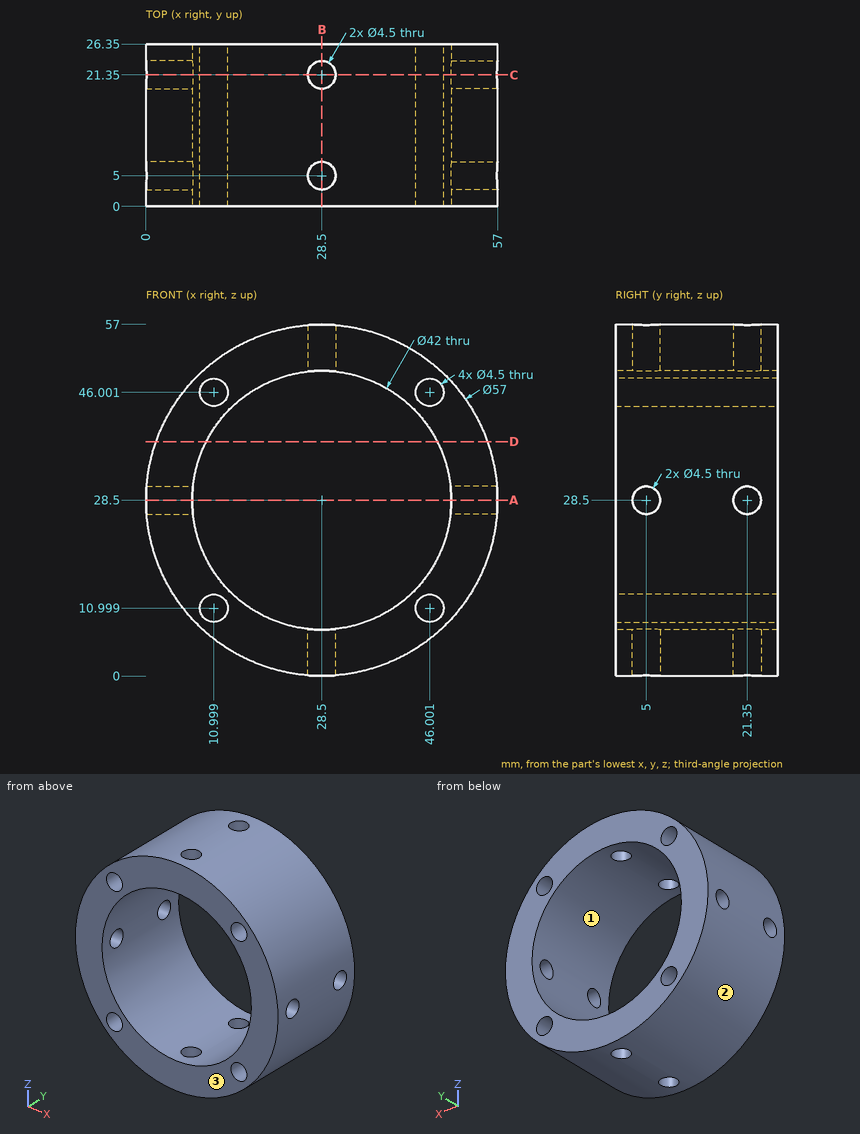
Here's the drawing with two shaded views (mm, measured from the low corner). I have some questions. Give positions to 0.01 mm unless a question says otherwise; leave off trailing zeros. Loops run counter-clockwise (first coordinate to the right, second up) from the corner with the lowest first, then second, coordinate; pieces in that order, holes last. Notation, with made-up numbers: M -17,35.25 L 6,35.25 A31 cw 6,70.25 Z; hole C -36.5,77.5 d1. An arc over 180 degrees is marked long. Use one line per item in the form item = value. Start each with the question number.
Q1. If we section it at B-B (x = 28.5): Write out the boundary of the cut face in (y, z).
Q2. If we section it at D-D (z = 38): Write out the boundary of the cut face in (x, y).
Q3. Will these pins go through, and if not, where does the flat tip stop? pin 1 Ø4 at (x, y) = (28.5, 5) entering from -Z; pin 2 Ø8 at (y, z) = (6, 8.5) entering from +X (3 decimals); pin 3 Ø1 at (x, y) = (37.5, 13) entering from +Z; pin 4 Ø1.5 at (x, y) = (47, 5) entering from -Z.
Q4. If we section it at C-C (y = 21.35): Write out the boundary of the cut face in (x, z).
Q5. I need wall thicknesses on line 1 along X through (y, z) = (1.5, 11) (1 decimal); line 2 along X through (y, z) = (14.75, 13); line 3 along Z through (x, y) = (12, 23) (1 decimal). Which ranges of each line are inside material? Lowest first, please.
Q6. Thinking about a two-plate mould opening in X: for the marked faces 1, 2 and 3, which applies, +X half, -X half, draft (parallel to the pull), parting line (faces both ways), or undercut?
Q7. If we section it at A-A (z = 28.5): Write out the boundary of the cut face in (x, y), then the cut area to 3 significant figures.
Taken from the geometry:
q1.outline = M 0,0 L 2.75,0 L 2.75,7.5 L 0,7.5 Z; M 0,49.5 L 2.75,49.5 L 2.75,57 L 0,57 Z; M 7.25,0 L 19.1,0 L 19.1,7.5 L 7.25,7.5 Z; M 7.25,49.5 L 19.1,49.5 L 19.1,57 L 7.25,57 Z; M 23.6,0 L 26.35,0 L 26.35,7.5 L 23.6,7.5 Z; M 23.6,49.5 L 26.35,49.5 L 26.35,57 L 23.6,57 Z
q2.outline = M 1.63,0 L 9.77,0 L 9.77,26.35 L 1.63,26.35 Z; M 47.23,0 L 55.37,0 L 55.37,26.35 L 47.23,26.35 Z
q3.pin_1 = through
q3.pin_2 = 52.085
q3.pin_3 = 55.7
q3.pin_4 = 6.2
q4.outline = M 0.09,26.25 A28.5 ccw 26.25,0.09 L 26.25,7.62 A21 cw 7.62,26.25 Z; M 0.09,30.75 L 7.62,30.75 A21 cw 26.25,49.38 L 26.25,56.91 A28.5 ccw Z; M 30.75,0.09 A28.5 ccw 56.91,26.25 L 49.38,26.25 A21 cw 30.75,7.62 Z; M 30.75,49.38 A21 cw 49.38,30.75 L 56.91,30.75 A28.5 ccw 30.75,56.91 Z; hole C 11,11 d4.5; hole C 11,46 d4.5; hole C 46,11 d4.5; hole C 46,46 d4.5
q5.line_1 = 6 to 8.7, 13.2 to 16.9, 40.1 to 43.8, 48.3 to 51
q5.line_2 = 4.58 to 9.97, 12.03 to 14.33, 42.67 to 44.97, 47.03 to 52.42
q5.line_3 = 5.3 to 9, 13 to 15.5, 41.5 to 44, 48 to 51.7
q6.face_1 = undercut
q6.face_2 = parting line
q6.face_3 = draft
q7.outline = M 0,0 L 7.5,0 L 7.5,2.75 L 0,2.75 Z; M 0,7.25 L 7.5,7.25 L 7.5,19.1 L 0,19.1 Z; M 0,23.6 L 7.5,23.6 L 7.5,26.35 L 0,26.35 Z; M 49.5,0 L 57,0 L 57,2.75 L 49.5,2.75 Z; M 49.5,7.25 L 57,7.25 L 57,19.1 L 49.5,19.1 Z; M 49.5,23.6 L 57,23.6 L 57,26.35 L 49.5,26.35 Z
q7.area = 260 mm^2
